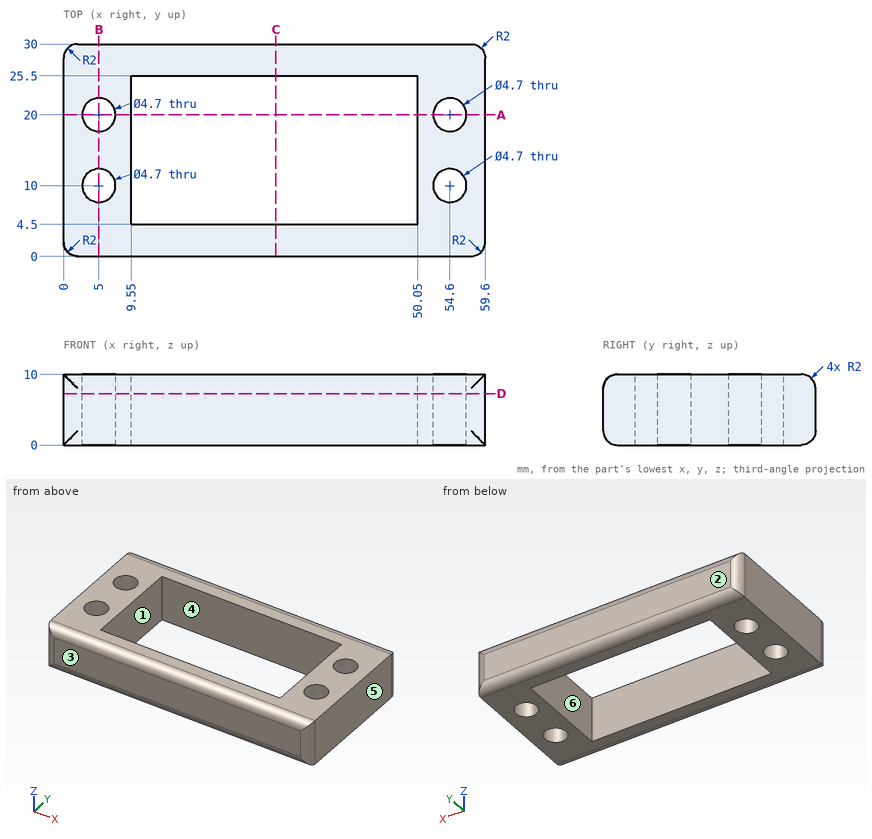
Input: dimensioned drawing with shaded views. Units: mm. Origin: part minimum x, y, z. A direction names the side the tool comes from. Give positions to 0.01 mm unless a question says otherwise; leave off trailing zeros. Write each loop counter-clockwise with the first axis right and the second up, starting at its lowest first coordinate (ties: lowest second). Pieces come first, ordered by that corner, then holes. Notation, with made-up numbers: (33, 89) -> (41, 89) arc R17 ccw to (41, 99) -> close; hole circle Ø8 at (17.25, 29.25). An arc over 180 degrees is marked (long way). Return JSON: item names as keys, results as strings. Group by question number.
1. Material intervals for line 1 (Y direction, x = 54.6, z = 7.75); line 2 (X direction, y = 10, z = 2.75); line 3 (X direction, y = 14.75, z = 9), sorted ascending. Write a range as from..to.
2. Section B-B, the plane x = 5. Output: boundary loops of the cut face in (y, z), then the cut area to 3 significant figures.
3. Section A-A, the plane y = 20. Output: boundary loops of the cut face in (x, z), then the cut area to 3 significant figures.
4. Section C-C, the plane x = 30. Output: boundary loops of the cut face in (y, z).
5. Access query for the marked faces 1 and 2. Directions: +Z, -Z, +X, -X, +Y, -Y. A direction counts if a zero-diameter tool reaches every point of the face in a straight line with its end or side. Return the directions, or none.
6. Mould query, pull axis Y, two halves, no side actions, for the marked faces 3, 4, 5 and 6. Classes: +Y half, -Y half, draft (parallel to the pull), parting line (faces both ways), or undercut.
7. Section D-D, the plane z = 7.25. Output: boundary loops of the cut face in (x, y), then the cut area to 3 significant figures.
Determined:
{
 "1": {"line 1": "y = 0..7.65, 12.35..17.65, 22.35..30", "line 2": "x = 0..2.65, 7.35..9.55, 50.05..52.25, 56.95..59.6", "line 3": "x = 0..9.55, 50.05..59.6"},
 "2": {"outline": "(0, 2) arc R2 ccw to (2, 0) -> (7.65, 0) -> (7.65, 10) -> (2, 10) arc R2 ccw to (0, 8) -> close; (12.35, 0) -> (17.65, 0) -> (17.65, 10) -> (12.35, 10) -> close; (22.35, 0) -> (28, 0) arc R2 ccw to (30, 2) -> (30, 8) arc R2 ccw to (28, 10) -> (22.35, 10) -> close", "area": "203 mm2"},
 "3": {"outline": "(0, 0) -> (2.65, 0) -> (2.65, 10) -> (0, 10) -> close; (7.35, 0) -> (9.55, 0) -> (9.55, 10) -> (7.35, 10) -> close; (50.05, 0) -> (52.25, 0) -> (52.25, 10) -> (50.05, 10) -> close; (56.95, 0) -> (59.6, 0) -> (59.6, 10) -> (56.95, 10) -> close", "area": "97.0 mm2"},
 "4": {"outline": "(0, 2) arc R2 ccw to (2, 0) -> (4.5, 0) -> (4.5, 10) -> (2, 10) arc R2 ccw to (0, 8) -> close; (25.5, 0) -> (28, 0) arc R2 ccw to (30, 2) -> (30, 8) arc R2 ccw to (28, 10) -> (25.5, 10) -> close"},
 "5": {"face 1": "+Z, -Z", "face 2": "+Z, -Z, +X, -X, +Y"},
 "6": {"face 3": "-Y half", "face 4": "undercut", "face 5": "draft", "face 6": "undercut"},
 "7": {"outline": "(0, 2) arc R2 ccw to (2, 0) -> (57.6, 0) arc R2 ccw to (59.6, 2) -> (59.6, 28) arc R2 ccw to (57.6, 30) -> (2, 30) arc R2 ccw to (0, 28) -> close; hole circle Ø4.7 at (5, 10); hole circle Ø4.7 at (5, 20); hole (9.55, 4.5) -> (50.05, 4.5) -> (50.05, 25.5) -> (9.55, 25.5) -> close; hole circle Ø4.7 at (54.6, 10); hole circle Ø4.7 at (54.6, 20)", "area": "865 mm2"}
}
